from build123d import *

# Parameters (mm, degrees)
BOSS_EXTRUDE1_START     = 26.5
SKETCH2_R               = 1.2
BOSS_EXTRUDE1_DEPTH     = 2
BOSS_EXTRUDE2_START     = -26.75
SKETCH3_R               = 4.5
BOSS_EXTRUDE2_DEPTH     = 5
CUT_EXTRUDE1_DEPTH      = 41.783728373
CUT_EXTRUDE1_DEPTH_BACK = 41.783728373
SKETCH4_R               = 2.95
BOSS_EXTRUDE3_START     = -4
SKETCH5_W               = 15
SKETCH5_H               = 5
BOSS_EXTRUDE3_DEPTH     = 4
BOSS_EXTRUDE6_START     = -26.75
SKETCH6_W               = 5.8
SKETCH6_H               = 4
BOSS_EXTRUDE6_DEPTH     = 45


with BuildPart() as part:
    # Sketch2 → Boss-Extrude1 (new body)
    with BuildSketch(Plane.XY.offset(-26.5).offset(BOSS_EXTRUDE1_START)):
        Polygon((-25, -17.75), (-20, -17.75), (-20, -26.75), (20, -26.75), (20, -17.75), (25, -17.75), (25, -31.75), (-25, -31.75), align=None)
        with Locations((22.5, -20.75)):
            Circle(SKETCH2_R, mode=Mode.SUBTRACT)
        with Locations((-22.5, -20.75)):
            Circle(SKETCH2_R, mode=Mode.SUBTRACT)
    extrude(amount=BOSS_EXTRUDE1_DEPTH)

    # Sketch3 → Boss-Extrude2 (add)
    with BuildSketch(Plane(origin=(0, 0, 0), x_dir=(1, 0, 0), z_dir=(0, 1, 0)).offset(BOSS_EXTRUDE2_START)):
        with Locations((0, -1)):
            Circle(SKETCH3_R)
    extrude(amount=-BOSS_EXTRUDE2_DEPTH)

    # Sketch4 → Cut-Extrude1 (cut, two sides: drawn at the far end of the back side and taken through both)
    with BuildSketch(Plane(origin=(0, 0, 0), x_dir=(1, 0, 0), z_dir=(0, 1, 0)).offset(-CUT_EXTRUDE1_DEPTH_BACK)):
        with Locations(Location((0, -1, 0), (0, 0, 270))):
            Circle(SKETCH4_R)
    extrude(amount=CUT_EXTRUDE1_DEPTH + CUT_EXTRUDE1_DEPTH_BACK, mode=Mode.SUBTRACT)

    # Sketch5 → Boss-Extrude3 (add)
    with BuildSketch(Plane.XY.offset(BOSS_EXTRUDE3_START)):
        with Locations((17.5, -29.25)):
            Rectangle(SKETCH5_W, SKETCH5_H)
        with Locations((-17.5, -29.25)):
            Rectangle(SKETCH5_W, SKETCH5_H)
    extrude(amount=BOSS_EXTRUDE3_DEPTH)

    # Sketch6 → Boss-Extrude6 (add)
    with BuildSketch(Plane(origin=(0, 0, 0), x_dir=(1, 0, 0), z_dir=(0, 1, 0)).offset(BOSS_EXTRUDE6_START)):
        with Locations((7.1, 2)):
            Rectangle(SKETCH6_W, SKETCH6_H)
        with Locations((-7.1, 2)):
            Rectangle(SKETCH6_W, SKETCH6_H)
    extrude(amount=-BOSS_EXTRUDE6_DEPTH)


solid = part.part
Geometry: final body of the model. Coordinates: model frame, mm. A direction names the side the tool comes from. Round coordinates to 2 decimals unless told otherwise and drop trailing zeros. Loops run counter-clockwise (first coordinate to the right, second up) from the corner with the lowest first, then second, coordinate; pieces in that order, holes last. Notation, with made-up numbers: (-3.5, -23.5) - (33.5, -23.5) arc R23 ccw to (33.5, -4.5) - close; hole circle Ø6 at (31.25, -39.5). An arc over 180 degrees is marked (long way). Write each question's results on one line, items separated by ' | '. Start each with the question number.
1) Cut plane B-B on y = -40.5. Return loops of the section in (x, z).
2) Mould query, pull axis Y, two halves, no side actions, for faces 1 (the face through (-23.45, -21.48, 0.99)), 2 (the face through (-0.3, -26.75, -2.5)), 3 (the face through (9.8, -43.9, -4)). Classes: released by +Y, released by -Y, zero draft, split by the parting line, or undercut.
3) Cut plane D-D on y = -20.75. Return loops of the section in (x, z), then the cut area to 3 significant figures.
4) Line query: probe 1 along X at (y, z) = (-28.1, 1); probe 2 along Y at (x, z) = (22.5, 0.9); probe 3 along X at (y, z) = (-41, -1.5). Output: solid intervals per line, ascending. Write a range as [from, to].
5) First-contact query: P1, Ø2, axis at y = -53, z = -1.5, coming from the -X side; P2, Ø5, axis at x = -5, z = 0, coming from the +Y side; P3, Ø3, axis at y = -52, z = -2.5, coming from the +X side. Flat tips, straight axial feed; report the tip coordinate or a pass-through.
6) Access query for faces 4 (the face through (17, -28, 2)), 5 (the face through (-10, -51, -2)), 6 (the face through (20, -22, 1)). Directions: +Z, -Z, +X, -X, +Y, -Y. A direction counts if a zero-diameter tool reaches every point of the face in a straight line with its end or side. Return the directions, or none.
7) Cut plane C-C on z = 1. Return loops of the section in (x, y).
8) Cut plane A-A on x = 22.5. Return loops of the section in (y, z).
Verdict:
1) outline: (-10, -4) - (-4.2, -4) - (-4.2, 0) - (-10, 0) - close; (4.2, -4) - (10, -4) - (10, 0) - (4.2, 0) - close
2) face 1: undercut | face 2: released by +Y | face 3: zero draft
3) outline: (-25, 0) - (-23.7, 0) - (-23.7, 2) - (-25, 2) - close; (-21.3, 0) - (-20, 0) - (-20, 2) - (-21.3, 2) - close; (20, 0) - (21.3, 0) - (21.3, 2) - (20, 2) - close; (23.7, 0) - (25, 0) - (25, 2) - (23.7, 2) - close | area: 10.4 mm2
4) probe 1: x = [-25, -2.95], [2.95, 25] | probe 2: y = [-31.75, -21.95], [-19.55, -17.75] | probe 3: x = [-10, -4.2], [4.2, 10]
5) P1: stops at x = -10 | P2: stops at y = -26.75 | P3: stops at x = 10
6) face 4: +Z, +X, +Y, -Y | face 5: +Z, -Z, -X, -Y | face 6: +Z, -Z, +Y
7) outline: (-25, -31.75) - (-2.95, -31.75) - (-2.95, -26.75) - (-20, -26.75) - (-20, -17.75) - (-25, -17.75) - close; (2.95, -31.75) - (25, -31.75) - (25, -17.75) - (20, -17.75) - (20, -26.75) - (2.95, -26.75) - close; hole circle Ø2.4 at (-22.5, -20.75); hole circle Ø2.4 at (22.5, -20.75)
8) outline: (-31.75, -4) - (-26.75, -4) - (-26.75, 0) - (-21.95, 0) - (-21.95, 2) - (-31.75, 2) - close; (-19.55, 0) - (-17.75, 0) - (-17.75, 2) - (-19.55, 2) - close
